```python
from build123d import *

# Parameters (mm, degrees)
EXTRUDE_1_DEPTH          = 76
EXTRUDE_2_DEPTH          = 2
EXTRUDE_2_DEPTH_BACK     = 76
EXTRUDE_3_DEPTH          = 9.5
CUT_EXTRUDE_1_DEPTH      = 78.5
CUT_EXTRUDE_2_DEPTH      = 4
CUT_EXTRUDE_2_DEPTH_BACK = 78.5
SKETCH_8_R               = 1
CUT_EXTRUDE_3_DEPTH      = 46.5
CUT_EXTRUDE_4_DEPTH      = 2


with BuildPart() as part:
    # Эскиз1 → Бобышка-Вытянуть1 (new body)
    with BuildSketch(Plane(origin=(0, 0, 0), x_dir=(1, 0, 0), z_dir=(0, 1, 0))):
        with BuildLine():
            Line((-13.5, -30.659419434), (-13.5, -31.749015733))
            ThreePointArc((-13.5, -31.749015733), (0, -34.5), (13.5, -31.749015733))
            Line((13.5, -31.749015733), (13.5, -30.659419434))
            ThreePointArc((13.5, -30.659419434), (12.013828707, -31.271679197), (10.5, -31.811947441))
            Line((10.5, -31.811947441), (10.5, -30.757112998))
            ThreePointArc((10.5, -30.757112998), (0, -32.5), (-10.5, -30.757112998))
            Line((-10.5, -30.757112998), (-10.5, -31.811947441))
            ThreePointArc((-10.5, -31.811947441), (-12.013828707, -31.271679197), (-13.5, -30.659419434))
        make_face()
    extrude(amount=EXTRUDE_1_DEPTH)

    # Эскиз2 → Бобышка-Вытянуть2 (add, two sides)
    with BuildSketch(Plane.XZ) as extrude_2_sk:
        with BuildLine():
            Line((-10.5, 31.811947441), (-10.5, 30.757112998))
            Line((-10.5, 30.757112998), (-10.5, 29.69848481))
            ThreePointArc((-10.5, 29.69848481), (0, 31.5), (10.5, 29.69848481))
            Line((10.5, 29.69848481), (10.5, 30.757112998))
            Line((10.5, 30.757112998), (10.5, 31.811947441))
            ThreePointArc((10.5, 31.811947441), (0, 33.5), (-10.5, 31.811947441))
        make_face()
    extrude(amount=EXTRUDE_2_DEPTH)
    extrude(extrude_2_sk.sketch, amount=-EXTRUDE_2_DEPTH_BACK)

    # Эскиз6 → Бобышка-Вытянуть3 (add)
    with BuildSketch(Plane(origin=(0, 76, 0), x_dir=(1, 0, 0), z_dir=(0, 1, 0))):
        with BuildLine():
            Line((-10.5, -30.757112998), (-10.5, -31.811947441))
            ThreePointArc((-10.5, -31.811947441), (-12.013828707, -31.271679197), (-13.5, -30.659419434))
            Line((-13.5, -30.659419434), (-13.5, -31.749015733))
            ThreePointArc((-13.5, -31.749015733), (0, -34.5), (13.5, -31.749015733))
            Line((13.5, -31.749015733), (13.5, -30.659419434))
            ThreePointArc((13.5, -30.659419434), (12.013828707, -31.271679197), (10.5, -31.811947441))
            Line((10.5, -31.811947441), (10.5, -30.757112998))
            ThreePointArc((10.5, -30.757112998), (0, -32.5), (-10.5, -30.757112998))
        make_face()
    extrude(amount=EXTRUDE_3_DEPTH)

    # Эскиз3 → Вырез-Вытянуть1 (cut)
    with BuildSketch(Plane.XY):
        with BuildLine():
            Line((-29.777002316, 76), (-29.777002316, 102.252406504))
            Line((-29.777002316, 102.252406504), (31.597845716, 102.252406504))
            Line((31.597845716, 102.252406504), (31.597845716, 75.705478865))
            Line((31.597845716, 75.705478865), (31.597845716, 73.652327708))
            Line((31.597845716, 73.652327708), (13.5, 73.652327708))
            ThreePointArc((13.5, 73.652327708), (12.995178699, 75.025430995), (11.721154976, 75.744542067))
            ThreePointArc((11.721154976, 75.744542067), (10.143272785, 76.524968738), (9.274814815, 78.056163941))
            ThreePointArc((9.274814815, 78.056163941), (0, 85.5), (-9.274814815, 78.056163941))
            ThreePointArc((-9.274814815, 78.056163941), (-10.143272784, 76.52496874), (-11.721154974, 75.744542071))
            ThreePointArc((-11.721154974, 75.744542071), (-12.995178698, 75.025430999), (-13.5, 73.652327712))
            Line((-13.5, 73.652327712), (-29.777002316, 73.652327712))
            Line((-29.777002316, 73.652327712), (-29.777002316, 76))
        make_face()
    extrude(amount=CUT_EXTRUDE_1_DEPTH, mode=Mode.SUBTRACT)

    # Эскиз7 → Вырез-Вытянуть2 (cut, two sides)
    with BuildSketch(Plane(origin=(0, 76, 0), x_dir=(-1, 0, 0), z_dir=(0, -1, 0))) as cut_extrude_2_sk:
        with BuildLine():
            Line((10.5, -29.69848481), (10.5, -31.811947441))
            ThreePointArc((10.5, -31.811947441), (0, -33.499999909), (-10.5, -31.811947441))
            Line((-10.5, -31.811947441), (-10.5, -29.69848481))
            ThreePointArc((-10.5, -29.69848481), (0, -31.5), (10.5, -29.69848481))
        make_face()
    extrude(amount=CUT_EXTRUDE_2_DEPTH, mode=Mode.SUBTRACT)
    extrude(cut_extrude_2_sk.sketch, amount=-CUT_EXTRUDE_2_DEPTH_BACK, mode=Mode.SUBTRACT)

    # Эскиз8 → Вырез-Вытянуть3 (cut)
    with BuildSketch(Plane.XY):
        with Locations((0, 81)):
            Circle(SKETCH_8_R)
    extrude(amount=CUT_EXTRUDE_3_DEPTH, mode=Mode.SUBTRACT)

    # Эскиз9 → Вырез-Вытянуть4 (cut)
    with BuildSketch(Plane.XZ.offset(2)):
        with BuildLine():
            Line((-10.5, 31.811947426), (-10.5, 30.755216126))
            ThreePointArc((-10.5, 30.755216126), (0, 32.500000073), (10.5, 30.755216126))
            Line((10.5, 30.755216126), (10.5, 31.811947441))
            ThreePointArc((10.5, 31.811947441), (-1e-09, 33.499999996), (-10.5, 31.811947426))
        make_face()
    extrude(amount=-CUT_EXTRUDE_4_DEPTH, mode=Mode.SUBTRACT)


solid = part.part
```
Design review of the part built by this model. Coordinates are the model's own, in mm. A direction names the side the tool comes from. Give positions to 0.01 mm unless a question says otherwise; leave off trailing zeros. Loops run counter-clockwise (first coordinate to the right, second up) from the corner with the lowest first, then second, coordinate; pieces in that order, holes last. Notation, with made-up numbers: M 23.25,57.5 L 44.25,57.5 A21 ccw 44.25,96.5 Z; hole C 52.25,78 d4. An arc over 180 degrees is marked long. Return JSON: item names as keys, results as strings. Group by question number.
Item 1: For probe 1 along Y at (x, z) = (0, 33.95); probe 2 along Y at (x, z) = (-0.75, 34.2); probe 3 along Y at (x, z) = (7.75, 33.05), list the stretches that pass through material, from the lowest coordinate up.
Item 2: We need section C-C (y = 10). Give the boundary of the cut face in (x, z), and give its area (3 significant figures).
Item 3: Tool access review of faces 5 (the flat face through (0, 0, 33)), 6 (the flat face through (0, -2, 32)), 7 (the flat face through (0, 72, 32)): name each direction out of +Z, -Z, +X, -X, +Y, -Y from which nothing blocks a thin tool from reaching the whole face with its end or side.
Item 4: Insertion check: pin 1 Ø1.6 at (x, y) = (0, 81) entering from +Z; pin 2 Ø2 at (x, y) = (-4.5, 49) entering from -Z; pin 3 Ø2 at (x, z) = (6.5, 32) entering from -Y; pin 4 Ø5 at (x, y) = (-3, 27.5) entering from +Z. Each pin has a flat end and moves straight along its axis. Give the tip position at first contact, or say it passes through.
Item 5: Mouldability with a two-part tool opening along X and no side actions: class faces 1 (the cylindrical face through (-0.1, 34.5, 31.5)), 2 (the cylindrical face through (-12.982, 75.041, 31.541)), 3 (the cylindrical face through (-0.2, 42.2, 34.5)), 4 (the cylindrical face through (13.01, 75.01, 31.54)) as released by +X, released by -X, zero draft, split by the parting line, or undercut.
Item 6: We need section A-A (x = 0). Give the boundary of the cut face in (y, z), and give its area (4 significant figures).
Item 7: We need section D-D (x = -3.5). Give the boundary of the cut face in (y, z).
Item 8: We need section B-B (y = 81). Give the boundary of the cut face in (x, z), and give its area (3 significant figures).
Output:
{
 "1": {"probe 1": "y = 0 to 80, 82 to 85.5", "probe 2": "y = 0 to 80.34, 81.66 to 85.47", "probe 3": "y = 0 to 81.49"},
 "2": {"outline": "M -13.5,30.66 A33.5 cw -10.5,31.81 L -10.5,29.7 A31.5 cw 10.5,29.7 L 10.5,31.81 A33.5 cw 13.5,30.66 L 13.5,31.75 A34.5 ccw -13.5,31.75 Z", "area": "70.5 mm^2"},
 "3": {"face 5": "+Z, -Y", "face 6": "+Z, -Z, +X, -X, -Y", "face 7": "-Z, +Y"},
 "4": {"pin 1": "passes through", "pin 2": "stops at z = 31.02", "pin 3": "stops at y = -2", "pin 4": "stops at z = 34.5"},
 "5": {"face 1": "undercut", "face 2": "released by -X", "face 3": "split by the parting line", "face 4": "released by +X"},
 "6": {"outline": "M -2,31.5 L 72,31.5 L 72,33.5 L 80,33.5 L 80,34.5 L 0,34.5 L 0,32.5 L -2,32.5 Z; M 82,33.5 L 85.5,33.5 L 85.5,34.5 L 82,34.5 Z", "area": "229.5 mm^2"},
 "7": {"outline": "M -2,31.3 L 72,31.3 L 72,33.32 L 84.83,33.32 L 84.83,34.32 L 0,34.32 L 0,32.31 L -2,32.31 Z"},
 "8": {"outline": "M -8.08,32.51 A33.5 cw -1,33.49 L -1,34.49 A34.5 ccw -8.08,33.54 Z; M 1,33.49 A33.5 cw 8.08,32.51 L 8.08,33.54 A34.5 ccw 1,34.49 Z", "area": "14.3 mm^2"}
}
